Check sheet for the drawn part. Datum: minimum x, y, z corner. Units: mm. Give positions to 0.01 mm unless a question says otherwise; leave off trailing zeros. Write each loop counter-clockwise with the first axis right and the second up, starting at its lowest first coordinate (ties: lowest second). Pieces come first, ordered by that corner, then holes. Notation, with made-up numbers: (-8, 78.5) - (50, 78.5) arc R6 ccw to (50, 86.5) - close; hole circle Ø5 at (54.5, 45). An arc over 180 degrees is marked (long way). Use a Markdown table: item, result.
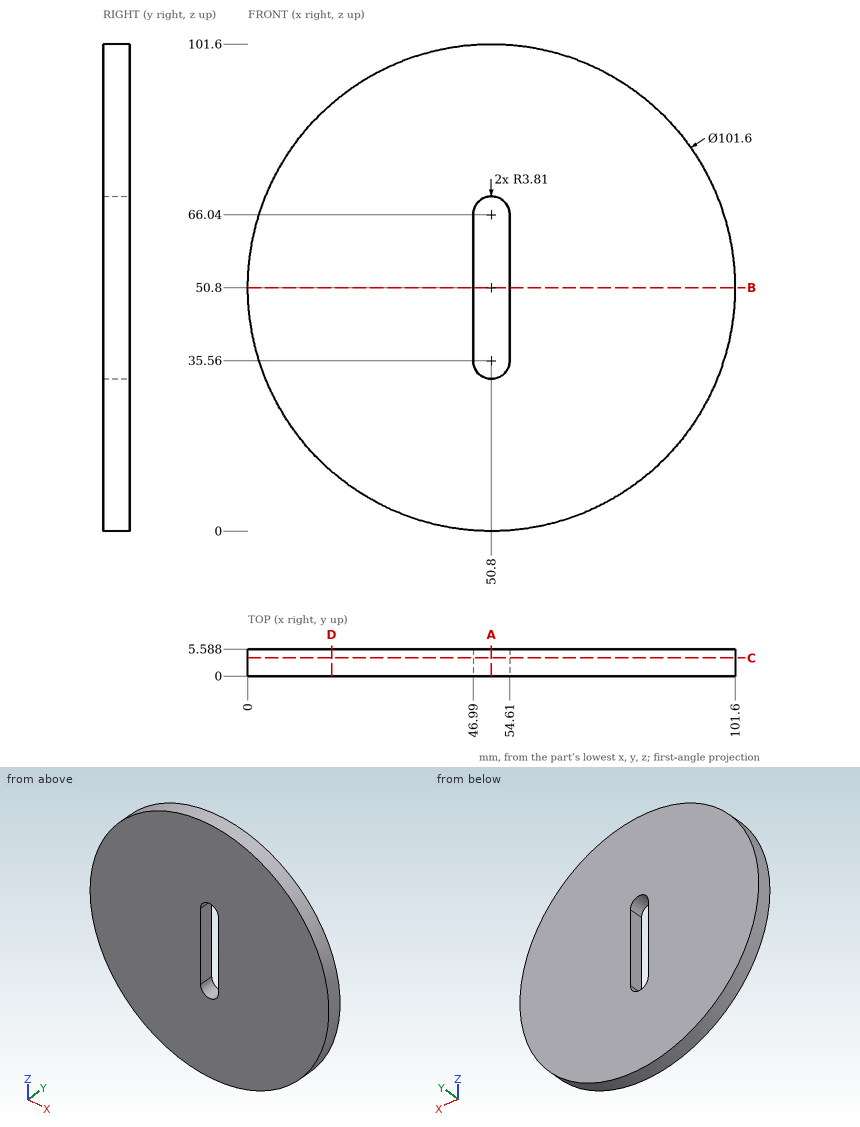
1) Depth check by flat-ended pin: P1, Ø1, axis at x = 28.5, y = 0.5, coming from the -Z side; P2, Ø2, axis at y = 4, z = 81.5, coming from the +X side; P3, Ø8, axis at x = 56.5, z = 63.5, coming from the -Y side. Enter the tip coordinate at first touch or a pass-through.
Working result:
| item | result |
|---|---|
| P1 | stops at z = 4.92 |
| P2 | stops at x = 92.01 |
| P3 | stops at y = 0 |
2) Material ranges on L1, parallel to Z at x = 50, y = 2.45; L2, parallel to X at y = 4, z = 61; L3, parallel to X at y = 5, z = 62, recorded low to high. Write a range as from..to.
Working result:
| item | result |
|---|---|
| L1 | z = 0.01..31.83, 69.77..101.59 |
| L2 | x = 1.03..46.99, 54.61..100.57 |
| L3 | x = 1.25..46.99, 54.61..100.35 |
3) Section check A-A on x = 50.8. Record the boundary of the cut face in (y, z).
Working result:
| item | result |
|---|---|
| outline | (0, 0) - (5.59, 0) - (5.59, 31.75) - (0, 31.75) - close; (0, 69.85) - (5.59, 69.85) - (5.59, 101.6) - (0, 101.6) - close |
4) Section check B-B on z = 50.8. Record the boundary of the cut face in (x, y), then the cut area to 3 significant figures.
Working result:
| item | result |
|---|---|
| outline | (0, 0) - (46.99, 0) - (46.99, 5.59) - (0, 5.59) - close; (54.61, 0) - (101.6, 0) - (101.6, 5.59) - (54.61, 5.59) - close |
| area | 525 mm² |
5) Section check C-C on y = 3.8. Record the boundary of the cut face in (x, z), then the cut area to 3 significant figures.
Working result:
| item | result |
|---|---|
| outline | circle Ø101.6 at (50.8, 50.8); hole (46.99, 35.56) arc R3.81 ccw to (54.61, 35.56) - (54.61, 66.04) arc R3.81 ccw to (46.99, 66.04) - close |
| area | 7,830 mm² |
6) Section check D-D on x = 17.5. Record the boundary of the cut face in (y, z), then the cut area to 3 significant figures.
Working result:
| item | result |
|---|---|
| outline | (0, 12.44) - (5.59, 12.44) - (5.59, 89.16) - (0, 89.16) - close |
| area | 429 mm² |
